from build123d import *

# Parameters (mm, degrees)
EXTRUDE1_DEPTH = 12.7
SKETCH2_R      = 4.7625
EXTRUDE2_DEPTH = 12.7


with BuildPart() as part:
    # Sketch1 → Extrude1 (new body)
    with BuildSketch(Plane(origin=(0, 0, 0), x_dir=(1, 0, 0), z_dir=(0, 1, 0))):
        Polygon((3.666174209, 6.35), (-3.666174209, 6.35), (-7.332348419, 0), (-3.666174209, -6.35), (3.666174209, -6.35), (7.332348419, 0), align=None)
    extrude(amount=EXTRUDE1_DEPTH)

    # Sketch2 → Extrude2 (add)
    with BuildSketch(Plane.XZ):
        with Locations(Location((0, 0, 0), (0, 0, 270))):
            Circle(SKETCH2_R)
    extrude(amount=EXTRUDE2_DEPTH)


solid = part.part
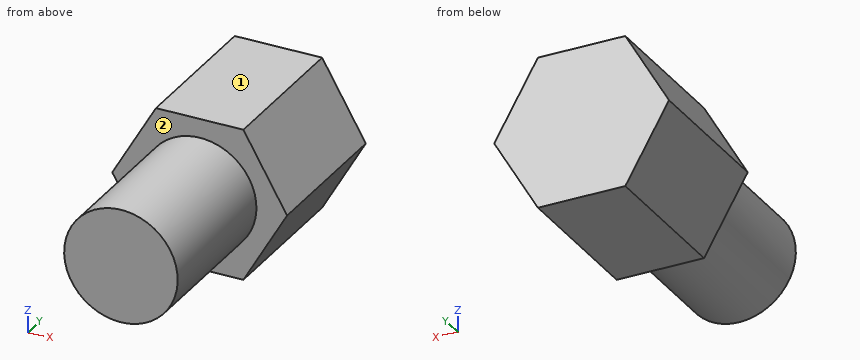
CAD build for the part. Positions are in the model's coordinates, mm. Face numbers are marked on the shaded views. A direction names the side the tool comes from. Coordinates: 2 decimals unless noted, no trailing zeros. Write each loop counter-clockwise with the first axis right and the second up, starting at its lowest first coordinate (ties: lowest second). Pieces come first, ordered by that corner, then holes. Notation, with made-up numbers: M 59,-21.75 L 70,-21.75 A29 ccw 70,0.25 Z; hole C -22.75,85 d1. An arc over 180 degrees is marked long. Answer as a JSON object with one key per item and string values. Group by question number.
1) Saw through at A-A (x = 0). Write the cut outline in (y, z), plus the area to 3 significant figures.
2) Saw through at C-C (z = -1.5). Write the cut outline in (x, y).
3) Tool access for the marked faces 1 and 2: list every direction of +Z, -Z, +X, -X, +Y, -Y with a clear straight run to the whole face (end or side of a thin tool).
4) Pin check, flat tips, straight feed: pin 1 Ø1.5 at (x, y) = (-2, -8.5) entering from -Z; pin 2 Ø1.5 at (x, z) = (-5.5, -4) entering from +Y; pin 3 Ø3 at (y, z) = (-10, 3) entering from -X. Stop position of each tip, or through.
5) Saw through at B-B (y = 3). Write the cut outline in (x, z).
6) Wall check: line 1 (Y direction, x = -0.5, z = 5); line 2 (X direction, y = -11, z = -3.75); line 3 (X direction, y = 11, z = 4.75). Give the ranges that are in metal, low to high. Write a range as from..to.
7) Saw through at D-D (y = -9.5). Write the cut outline in (x, z) (1 decimal).
Values follow:
{
 "1": {"outline": "M -12.7,-4.76 L 0,-4.76 L 0,-6.35 L 12.7,-6.35 L 12.7,6.35 L 0,6.35 L 0,4.76 L -12.7,4.76 Z", "area": "282 mm2"},
 "2": {"outline": "M -6.47,0 L -4.52,0 L -4.52,-12.7 L 4.52,-12.7 L 4.52,0 L 6.47,0 L 6.47,12.7 L -6.47,12.7 Z"},
 "3": {"face 1": "+Z, +X, -X, +Y, -Y", "face 2": "-Y"},
 "4": {"pin 1": "stops at z = -4.6", "pin 2": "stops at y = 12.7", "pin 3": "stops at x = -4.52"},
 "5": {"outline": "M -7.33,0 L -3.67,-6.35 L 3.67,-6.35 L 7.33,0 L 3.67,6.35 L -3.67,6.35 Z"},
 "6": {"line 1": "y = 0..12.7", "line 2": "x = -2.94..2.94", "line 3": "x = -4.59..4.59"},
 "7": {"outline": "C 0,0 d9.5"}
}
